from build123d import *

# Parameters (mm, degrees)
EXTRUDE_1_DEPTH = 20
SKETCH_2_R      = 30
EXTRUDE_2_DEPTH = 5
SKETCH_3_R      = 30
EXTRUDE_3_DEPTH = 5


with BuildPart() as part:
    # 草图1 → 凸台-拉伸1 (new body)
    with BuildSketch(Plane(origin=(0, 0, 0), x_dir=(0, 0, -1), z_dir=(1, 0, 0))):
        with BuildLine():
            Line((0, 30), (300, 30))
            ThreePointArc((300, 30), (330, 0), (300, -30))
            Line((300, -30), (0, -30))
            ThreePointArc((0, -30), (-30, 0), (0, 30))
        make_face()
    extrude(amount=EXTRUDE_1_DEPTH)

    # 草图2 → 凸台-拉伸2 (add)
    with BuildSketch(Plane(origin=(20, 0, 0), x_dir=(0, 0, -1), z_dir=(1, 0, 0))):
        with Locations(Location((300, 0, 0), (0, 0, 90))):
            Circle(SKETCH_2_R)
    extrude(amount=EXTRUDE_2_DEPTH)

    # 草图3 → 凸台-拉伸3 (add)
    with BuildSketch(Plane.ZY):
        Circle(SKETCH_3_R)
    extrude(amount=EXTRUDE_3_DEPTH)


solid = part.part
The listing builds one solid part. Answer for the finished solid, in the listing's coordinates (mm). A direction names the side the tool comes from. Give positions to 0.01 mm unless a question says otherwise; leave off trailing zeros. Order: outer loops, then holes, each group sorted by start corner. A loop starts at its lowest first (then second) coordinate and runs counter-clockwise, first axis right, second up. Notation, with made-up numbers: (85.5, 61) - (130.5, 61) arc R8 cw to (130.5, 69) - close; hole circle Ø10 at (0, 15). An arc over 180 degrees is marked (long way). Answer as CSV lines item,"result".
Q1. A cutting plane is placed at C-C, the plane x = 7. Determine the outline of the cut face in (y, z).
Answer key:
outline,"(-30, -300) arc R30 ccw to (30, -300) - (30, 0) arc R30 ccw to (-30, 0) - close"
Q2. A cutting plane is placed at D-D, the plane z = -134. Determine the outline of the cut face in (x, y).
Answer key:
outline,"(0, -30) - (20, -30) - (20, 30) - (0, 30) - close"
Q3. Each of these flat-tipped pins is pushed along its axis until it touches: pin 1 Ø10 at (x, y) = (2.5, -13.5) entering from +Z; pin 2 Ø10 at (x, y) = (5, -9) entering from -Z; pin 3 Ø1 at (x, y) = (11, 17.5) entering from -Z. Where does it stop, or does it pass through?
Answer key:
pin 1,"stops at z = 28.77"
pin 2,"stops at z = -329.73"
pin 3,"stops at z = -324.72"
Q4. A cutting plane is placed at A-A, the plane y = 0. Determine the outline of the cut face in (x, z), and give its area (3 significant figures).
Answer key:
outline,"(-5, -30) - (0, -30) - (0, -330) - (25, -330) - (25, -270) - (20, -270) - (20, 30) - (-5, 30) - close"
area,"7,800 mm^2"
Q5. Straight lines are drawn through the part: L1, parallel to X at y = 15, z = -268; L2, parallel to X at y = 27, z = -313; L3, parallel to Z at x = 17.75, y = 2. For each, find the intervals that lie inside material, in ascending order.
Answer key:
L1,"x = 0 to 20"
L2,"x = 0 to 25"
L3,"z = -329.93 to 29.93"
Q6. A cutting plane is placed at B-B, the plane z = -292. Determine the outline of the cut face in (x, y).
Answer key:
outline,"(0, -30) - (20, -30) - (20, -28.91) - (25, -28.91) - (25, 28.91) - (20, 28.91) - (20, 30) - (0, 30) - close"
Q7. Which of the six approach directions +Z, -Z, +X, -X, +Y, -Y give full straight-line access (tool end or side, diameter ignored) to faces 1 (the face through (15.103, -6.503, -329.287)), 2 (the face through (10, -30, -152))?
Answer key:
face 1,"+X"
face 2,"+Z, -Z, +X, -X, -Y"
